from build123d import *

# Parameters (mm, degrees)
SKETCH1_R           = 7.5
BOSS_EXTRUDE1_DEPTH = 6
CHAMFER1_SIZE       = 0.5
SKETCH2_R           = 1.25
CUT_EXTRUDE1_DEPTH  = 10


with BuildPart() as part:
    # Sketch1 → Boss-Extrude1 (new body)
    with BuildSketch(Plane.XY):
        with BuildLine():
            Line((9.643002644, -1.05), (13.943002644, -1.05))
            Line((13.943002644, -1.05), (13.943002644, 1.05))
            Line((13.943002644, 1.05), (9.643002644, 1.05))
            ThreePointArc((9.643002644, 1.05), (0, 9.7), (-9.643002644, 1.05))
            Line((-9.643002644, 1.05), (-13.943002644, 1.05))
            Line((-13.943002644, 1.05), (-13.943002644, -1.05))
            Line((-13.943002644, -1.05), (-9.643002644, -1.05))
            ThreePointArc((-9.643002644, -1.05), (0, -9.7), (9.643002644, -1.05))
        make_face()
        Circle(SKETCH1_R, mode=Mode.SUBTRACT)
    extrude(amount=BOSS_EXTRUDE1_DEPTH)

    # Chamfer1
    chamfer1_edges = [part.edges().sort_by_distance(p)[0] for p in [
        (0, -9.7, 0),
        (-11.793002644, -1.05, 0),
        (-13.943002644, 0, 0),
        (-11.793002644, 1.05, 0),
        (-11.793002644, -1.05, 6),
        (0, -9.7, 6),
        (11.793002644, -1.05, 6),
        (-7.5, 0, 0),
        (-7.5, 0, 6),
        (13.943002644, 0, 6),
        (11.793002644, 1.05, 6),
        (0, 9.7, 6),
        (-11.793002644, 1.05, 6),
        (0, 9.7, 0),
        (-13.943002644, 0, 6),
        (11.793002644, 1.05, 0),
        (13.943002644, 0, 0),
        (11.793002644, -1.05, 0),
    ]]
    chamfer(chamfer1_edges, length=CHAMFER1_SIZE)

    # Sketch2 → Cut-Extrude1 (cut)
    with BuildSketch(Plane(origin=(0, 0, 0), x_dir=(-1, 0, 0), z_dir=(0, 0, -1))):
        with Locations((0, 7.5)):
            Circle(SKETCH2_R)
    extrude(amount=-CUT_EXTRUDE1_DEPTH, mode=Mode.SUBTRACT)


solid = part.part
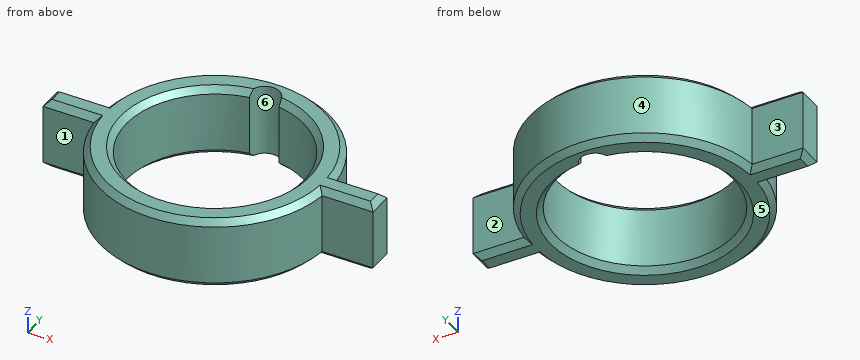
Source: CAD feature listing. Evaluate the final solid. Frame: model axes, mm. Face numbers are marked on the shaded views. A direction names the side the tool comes from. Give positions to 0.01 mm unless a question says otherwise; leave off trailing zeros. Loops run counter-clockwise (first coordinate to the right, second up) from the corner with the lowest first, then second, coordinate; pieces in that order, holes last. Notation, with made-up numbers: (-14, 82) -> (-2, 82) arc R16 cw to (-2, 106) -> close; hole circle Ø8 at (51, 57.5). An arc over 180 degrees is marked (long way). Use a Markdown table: item, result. Add a question column.
1) Section query D-D, the plane z = 1.5. Return the cut outline in (x, y), then the cut area to 3 significant figures.
2) Section query C-C, the plane x = 10.25. Return the cut outline in (y, z).
3) Line query: line 1 along X through (y, z) = (1.75, 1); line 2 along Y through (x, z) = (11, 3.75); line 3 along X through (y, z) = (0, 1.65). Output: solid intervals per line, ascending. Write a range as [from, to].
4) First-contact query: pin 1 (3 mm diameter, centred on x = 4.5, y = -4.5, fed in from +Z); pin 2 (1.3 mm diameter, centred on x = 12.5, z = 2, fed in from +Y); pin 3 (1 mm diameter, centred on x = -1, z = 2.5, fed in from -Y); pin 4 (2 mm diameter, centred on x = 0, y = 7.5, fed in from -Z). Flat tips, straight axial feed; report the tip coordinate or a pass-through.
5) Reachability of the marked faces 1, 2 and 3 from +Z, -Z, +X, -X, +Y, -Y: full face, straight path, thin tool, end or side. Return the list, or none.
6) Pull-direction query (X, two-part tool) for the marked faces 4, 5 and 6; classes: +X half, -X half, draft (parallel to the pull), parting line (faces both ways), or undercut.
7) Section query A-A, the plane x = 0. Return the cut outline in (y, z).
8) Section query B-B, the plane y = 0. Return the cut outline in (x, z), then the cut area to 3 significant figures.
Numbers:
| question | item | result |
|---|---|---|
| 1 | outline | (-13.94, -1.05) -> (-9.64, -1.05) arc R9.7 ccw to (9.64, -1.05) -> (13.94, -1.05) -> (13.94, 1.05) -> (9.64, 1.05) arc R9.7 ccw to (-9.64, 1.05) -> (-13.94, 1.05) -> close; hole (-1.25, 7.4) arc R7.5 ccw (long way) to (1.25, 7.4) arc R1.25 ccw (long way) to start |
| 1 | area | 134 mm2 |
| 2 | outline | (-1.05, 0.5) -> (-0.55, 0) -> (0.55, 0) -> (1.05, 0.5) -> (1.05, 5.5) -> (0.55, 6) -> (-0.55, 6) -> (-1.05, 5.5) -> close |
| 3 | line 1 | x = [-9.54, -7.29], [7.29, 9.54] |
| 3 | line 2 | y = [-1.05, 1.05] |
| 3 | line 3 | x = [-13.94, -7.5], [7.5, 13.94] |
| 4 | pin 1 | stops at z = 5.86 |
| 4 | pin 2 | stops at y = 1.05 |
| 4 | pin 3 | stops at y = -9.69 |
| 4 | pin 4 | passes through |
| 5 | face 1 | +Z, -Z, -X, -Y |
| 5 | face 2 | +Z, -Z, +X, +Y |
| 5 | face 3 | +Z, -Z, -X, +Y |
| 6 | face 4 | parting line |
| 6 | face 5 | draft |
| 6 | face 6 | undercut |
| 7 | outline | (-9.7, 0.5) -> (-9.2, 0) -> (-8, 0) -> (-7.5, 0.5) -> (-7.5, 5.5) -> (-8, 6) -> (-9.2, 6) -> (-9.7, 5.5) -> close; (8.75, 0) -> (9.2, 0) -> (9.7, 0.5) -> (9.7, 5.5) -> (9.2, 6) -> (8.75, 6) -> close |
| 8 | outline | (-13.94, 0.5) -> (-13.44, 0) -> (-8, 0) -> (-7.5, 0.5) -> (-7.5, 5.5) -> (-8, 6) -> (-13.44, 6) -> (-13.94, 5.5) -> close; (7.5, 0.5) -> (8, 0) -> (13.44, 0) -> (13.94, 0.5) -> (13.94, 5.5) -> (13.44, 6) -> (8, 6) -> (7.5, 5.5) -> close |
| 8 | area | 76.3 mm2 |
